Input: part model. Units: mm. Frame: model coordinates. A direction names the side the tool comes from. Round coordinates to 2 decimals unless told otherwise and drop trailing zeros. Loops run counter-clockwise (first coordinate to the right, second up) from the corner with the lowest first, then second, coordinate; pieces in that order, holes last. Notation, with made-up numbers: M 36,47 L 44,47 A15 ccw 44,57 Z; hole C -34,-9.75 d6. An arc over 180 degrees is marked long. Return JSON: item names as keys, results as strings. Group by question number.
1) Section D-D (y = 24.5). Output: boundary loops of the cut face in (x, z), plus the area to 3 significant figures.
2) Contact query for flat-ended pins moving along their axis: P1, Ø4.5, axis at x = -27.5, z = 21.5, coming from the +Y side; P2, Ø22.5, axis at x = -7, y = 9.5, coming from the +Z side; P3, Ø12, axis at x = 29, y = 0, coming from the +Z side. Output: stop coordinate, or through.
3) Access query for faces 1 (the face through (0, 8, 0)), 2 (the face through (0, -30.05, 18)), 3 (the face through (-26, 0, 28)), 4 (the face through (18.5, 0, 23)). Directions: +Z, -Z, +X, -X, +Y, -Y. A direction counts if a zero-diameter tool reaches every point of the face in a straight line with its end or side. Return the directions, or none.
4) Section B-B (x = -24). Output: boundary loops of the cut face in (y, z), plus the area to 3 significant figures.
5) Material intervals for line 1 (X direction, y = -15, z = 26.5); line 2 (Z direction, x = 27.5, y = -12); line 3 (Y direction, x = -22, z = 12), sorted ascending. Write a range as from..to.
6) Section C-C (z = 26). Output: boundary loops of the cut face in (x, y).
7) Mould query, pull axis Z, two halves, no side actions, for faces 5 (the face through (0, 0, -4)), 6 (the face through (-18.5, 0, 23)), 7 (the face through (0, -22, 41.1)), 8 (the face through (26, 0, 19)). Classes: +Z half, -Z half, draft (parallel to the pull), parting line (faces both ways), or undercut.
8) Section A-A (y = -5.5). Output: boundary loops of the cut face in (x, z), plus the area to 3 significant figures.
from build123d import *

# Parameters (mm, degrees)
F0_W     = 37
F0_H     = 30.1
F0_H_2   = 15
F0_W_2   = 15
F1_DEPTH = 4
F2_DEPTH = 41.1
F3_W     = 15
F3_H     = 9
F4_DEPTH = 30.1


with BuildPart() as f1:
    # F0 (on Top) → F1 (new body)
    with BuildSketch(Plane.XY):
        Polygon((33.5, -15.05), (33.5, 30.05), (-33.5, 30.05), (-33.5, -15.05), (-18.5, -15.05), (-18.5, 15.05), (18.5, 15.05), (18.5, -15.05), align=None)
        Rectangle(F0_W, F0_H)
        with Locations((0, -22.55)):
            Rectangle(F0_W, F0_H_2)
        with Locations((-26, -22.55)):
            Rectangle(F0_W_2, F0_H_2)
        with Locations((26, -22.55)):
            Rectangle(F0_W_2, F0_H_2)
    extrude(amount=-F1_DEPTH)

    # F0 (on Top) → F2 (join)
    with BuildSketch(Plane.XY):
        with Locations((0, -22.55)):
            Rectangle(F0_W, F0_H_2)
        with Locations((-26, -22.55)):
            Rectangle(F0_W_2, F0_H_2)
        with Locations((26, -22.55)):
            Rectangle(F0_W_2, F0_H_2)
    extrude(amount=F2_DEPTH)

    # F3 (on face) → F4 (join)
    with BuildSketch(Plane(origin=(0, -15.05, 0), x_dir=(-1, 0, 0), z_dir=(0, 1, 0))):
        with Locations((26, 23.5)):
            Rectangle(F3_W, F3_H)
        with Locations((-26, 23.5)):
            Rectangle(F3_W, F3_H)
    extrude(amount=F4_DEPTH)


solid = f1.part
Returned:
{
 "1": {"outline": "M -33.5,-4 L 33.5,-4 L 33.5,0 L -33.5,0 Z", "area": "268 mm^2"},
 "2": {"P1": "stops at y = 15.05", "P2": "stops at z = 0", "P3": "stops at z = 28"},
 "3": {"face 1": "+X, -X, +Y", "face 2": "+Z, -Z, +X, -X, -Y", "face 3": "+Z, +X, -X, +Y", "face 4": "+Z, +Y"},
 "4": {"outline": "M -30.05,-4 L 30.05,-4 L 30.05,0 L -15.05,0 L -15.05,19 L 15.05,19 L 15.05,28 L -15.05,28 L -15.05,41.1 L -30.05,41.1 Z", "area": "1,130 mm^2"},
 "5": {"line 1": "x = -33.5..-18.5, 18.5..33.5", "line 2": "z = -4..0, 19..28", "line 3": "y = -30.05..-15.05"},
 "6": {"outline": "M -33.5,-30.05 L 33.5,-30.05 L 33.5,15.05 L 18.5,15.05 L 18.5,-15.05 L -18.5,-15.05 L -18.5,15.05 L -33.5,15.05 Z"},
 "7": {"face 5": "-Z half", "face 6": "draft", "face 7": "+Z half", "face 8": "undercut"},
 "8": {"outline": "M -33.5,-4 L 33.5,-4 L 33.5,0 L -33.5,0 Z; M -33.5,19 L -18.5,19 L -18.5,28 L -33.5,28 Z; M 18.5,19 L 33.5,19 L 33.5,28 L 18.5,28 Z", "area": "538 mm^2"}
}
